from build123d import *

# Parameters (mm, degrees)
F0_W        = 127
F0_H        = 76.2
F1_DEPTH    = 76.2
F2_R        = 12.7
F3_DEPTH    = 76.201
F4_R        = 5.08
F5_T1_DEPTH = 91.44
F6_T1_DEPTH = 92.1682991577


# Not quite as in the source:
# - a fillet or chamfer that OpenCascade refuses, or shapes differently, is made with other operations: its cross-section is extruded or revolved along the edge and cut away or added


with BuildPart() as f1:
    # F0 (on Front) → F1 (new body)
    with BuildSketch(Plane.XZ):
        with Locations((1.319276005, 11.0456193745)):
            Rectangle(F0_W, F0_H)
    extrude(amount=F1_DEPTH)

    # F2 (on face) → F3 (cut, through all)
    with BuildSketch(Plane.XY.offset(49.1456193745)):
        with Locations((0, -38.1)):
            Circle(F2_R)
    extrude(amount=-F3_DEPTH, mode=Mode.SUBTRACT)

    # F4
    f4_edges = [f1.edges().sort_by_distance(p)[0] for p in [
        (64.819276, -38.1, 49.145619),
        (1.319276, 0, 49.145619),
        (1.319276, -76.2, 49.145619),
        (-62.180724, -38.1, 49.145619),
        (-12.7, -38.1, 49.145619),
        (-62.180724, -38.1, -27.054381),
        (1.319276, 0, -27.054381),
        (1.319276, -76.2, -27.054381),
        (64.819276, -38.1, -27.054381),
        (-12.7, -38.1, -27.054381),
    ]]
    fillet(f4_edges, radius=F4_R)

    # F5: fillet of radius 5.08 on 4 edges, made by hand

    # F5_s2 → F5_t1 (cut)
    with BuildSketch(Plane.XY.offset(-34.6743806255)):
        with BuildLine():
            ThreePointArc((-57.100723995, 0), (-60.6928264434, -1.4878975516), (-62.180723995, -5.08))
            Line((-62.180723995, -5.08), (-62.180723995, 0))
            Line((-62.180723995, 0), (-57.100723995, 0))
        make_face()
        with BuildLine():
            ThreePointArc((-57.100723995, -76.2), (-60.6928264434, -74.7121024484), (-62.180723995, -71.12))
            Line((-62.180723995, -71.12), (-62.180723995, -76.2))
            Line((-62.180723995, -76.2), (-57.100723995, -76.2))
        make_face()
    extrude(amount=F5_T1_DEPTH, mode=Mode.SUBTRACT)

    # F6: chamfer of 5.08 on 4 edges, made by hand

    # F6_s2 → F6_t1 (cut)
    with BuildSketch(Plane.XY.offset(-35.0385302044)):
        Polygon((64.819276005, -5.08), (59.739276005, 0), (64.819276005, 0), align=None)
        Polygon((64.819276005, -71.12), (59.739276005, -76.2), (64.819276005, -76.2), align=None)
    extrude(amount=F6_T1_DEPTH, mode=Mode.SUBTRACT)


solid = f1.part
Part model, mm, in its own coordinate system. Coordinates: 2 decimals unless noted, no trailing zeros. Loops run counter-clockwise (first coordinate to the right, second up) from the corner with the lowest first, then second, coordinate; pieces in that order, holes last. Notation, with made-up numbers: M 24,39 L 83,39 A16 ccw 83,43 Z; hole C 62.5,-9 d2. An arc over 180 degrees is marked long. Use a Markdown table: item, result. Add a question column.
Q1. Probe L1, parallel to X at y = -38, z = 14; L2, parallel to Y at x = 0, z = -5.5; L3, parallel to Y at x = -6.5, z = -16.5. List the from-to ranges inside material, lowest first.
Q2. Cut at A-A (y = -38.1). Write the cut outline in (x, z).
Q3. Cut at B-B (z = -14.5). Write the cut outline in (x, y), and give its area (3 significant figures).
Q4. Cut at C-C (x = 0). Write the cut outline in (y, z), and give its area (3 significant figures).
Q5. Mould opens along X. For faces 1 (the cylindrical face through (-60.73, -38.61, -25.53)), 2 (the flat face through (1, 0, 12)), 3 (the cylindrical face through (-2.75, -50.5, 11.51)) say: +X half, -X half, draft (parallel to the pull), parting line (faces both ways), or undercut.
Worked out:
| question | item | result |
|---|---|---|
| 1 | L1 | x = -62.18 to -12.7, 12.7 to 64.82 |
| 1 | L2 | y = -76.2 to -50.8, -25.4 to 0 |
| 1 | L3 | y = -76.2 to -49.01, -27.19 to 0 |
| 2 | outline | M -62.18,-21.97 A5.08 ccw -57.1,-27.05 L -17.78,-27.05 A5.08 ccw -12.7,-21.97 L -12.7,44.07 A5.08 ccw -17.78,49.15 L -57.1,49.15 A5.08 ccw -62.18,44.07 Z; M 12.7,-21.97 A5.08 ccw 17.78,-27.05 L 59.74,-27.05 A5.08 ccw 64.82,-21.97 L 64.82,44.07 A5.08 ccw 59.74,49.15 L 17.78,49.15 A5.08 ccw 12.7,44.07 Z |
| 3 | outline | M -62.18,-71.12 A5.08 ccw -57.1,-76.2 L 59.74,-76.2 L 64.82,-71.12 L 64.82,-5.08 L 59.74,0 L -57.1,0 A5.08 ccw -62.18,-5.08 Z; hole C 0,-38.1 d25.4 |
| 3 | area | 9,130 mm2 |
| 4 | outline | M -76.2,-21.97 A5.08 ccw -71.12,-27.05 L -55.88,-27.05 A5.08 ccw -50.8,-21.97 L -50.8,44.07 A5.08 ccw -55.88,49.15 L -71.12,49.15 A5.08 ccw -76.2,44.07 Z; M -25.4,-21.97 A5.08 ccw -20.32,-27.05 L -5.08,-27.05 A5.08 ccw 0,-21.97 L 0,44.07 A5.08 ccw -5.08,49.15 L -20.32,49.15 A5.08 ccw -25.4,44.07 Z |
| 4 | area | 3,830 mm2 |
| 5 | face 1 | -X half |
| 5 | face 2 | draft |
| 5 | face 3 | undercut |
